```python
from build123d import *

# Parameters (mm, degrees)
EXTRUDE_1_DEPTH       = 2
HOLE_WIZARD_M81_D     = 8.4
HOLE_WIZARD_M81_DEPTH = 2
CHAMFER_1_SIZE        = 2


with BuildPart() as part:
    # Эскиз1 → Бобышка-Вытянуть1 (new body)
    with BuildSketch(Plane(origin=(0, 0, 0), x_dir=(1, 0, 0), z_dir=(0, 0, -1))):
        Polygon((0, 0), (0, 200), (100, 200), (100, 100), (50, 0), align=None)
    extrude(amount=EXTRUDE_1_DEPTH)

    # Отверстие с зазором M81
    with Locations(Plane(origin=(0, 0, -2), x_dir=(1, 0, 0), z_dir=(0, 0, -1))):
        with Locations((25, 175), (25, 125), (25, 75), (25, 25), (75, 175), (75, 125)):
            Hole(HOLE_WIZARD_M81_D / 2, depth=HOLE_WIZARD_M81_DEPTH)

    # Фаска1
    chamfer_1_edges = [part.edges().sort_by_distance(p)[0] for p in [
        (0, 0, -1),
        (0, -200, -1),
        (100, -200, -1),
    ]]
    chamfer(chamfer_1_edges, length=CHAMFER_1_SIZE)


solid = part.part
```
The model under review builds one solid part; all positions refer to its coordinate system, in mm. Round coordinates to 2 decimals unless told otherwise and drop trailing zeros. Loops run counter-clockwise (first coordinate to the right, second up) from the corner with the lowest first, then second, coordinate; pieces in that order, holes last. Notation, with made-up numbers: (47.5, 48.25) - (78.5, 48.25) arc R15 cw to (78.5, 65.25) - close; hole circle Ø5 at (71.5, -4.75). An arc over 180 degrees is marked (long way). Write each question's results on one line, items separated by ' | '. Start each with the question number.
Q1. Draft analysis for pull direction X (two halves, no side actions). For faces 1 (the flat face through (75.35, -50.7, -0.99)), 2 (the cylindrical face through (25.91, -70.9, -0.99)), 3 (the flat face through (51, -101, -2)), 4 (the cylindrical face through (28.3, -122.4, -1)), state which applies: pulls with the +X half, pulls with the -X half, needs draft (parallel to the pull), parting line crosses it, or undercut.
Q2. Take a section at C-C on x = 75. Give the boundary of the cut face in (y, z), plus the area to 3 significant figures.
Q3. Take a section at B-B on y = -175. Give the boundary of the cut face in (x, z), plus the area to 3 significant figures.
Q4. Wall thickness on line 1 along Y through (x, z) = (25, -0.2); line 2 along X through (y, z) = (-175, -1.5); line 3 along Y through (x, z) = (75, -1): over which ranges is each line inside the solid? List them lowest first. Write a range as [from, to].
Q5. Insertion check: P1, Ø5, axis at x = 25, y = -175, coming from the +Z side. The pin has a flat end and moves straight along its axis. Give the tip position at first contact, or say it passes through.
Q6. Take a section at D-D on y = -25. Give the boundary of the cut face in (x, z), plus the area to 3 significant figures.
Q7. Take a section at A-A on x = 25. Give the boundary of the cut face in (y, z).
Data:
1) face 1: pulls with the +X half | face 2: undercut | face 3: needs draft | face 4: undercut
2) outline: (-200, -2) - (-179.2, -2) - (-179.2, 0) - (-200, 0) - close; (-170.8, -2) - (-129.2, -2) - (-129.2, 0) - (-170.8, 0) - close; (-120.8, -2) - (-50, -2) - (-50, 0) - (-120.8, 0) - close | area: 266 mm²
3) outline: (0, -2) - (20.8, -2) - (20.8, 0) - (0, 0) - close; (29.2, -2) - (70.8, -2) - (70.8, 0) - (29.2, 0) - close; (79.2, -2) - (100, -2) - (100, 0) - (79.2, 0) - close | area: 166 mm²
4) line 1: y = [-200, -179.2], [-170.8, -129.2], [-120.8, -79.2], [-70.8, -29.2], [-20.8, 0] | line 2: x = [0, 20.8], [29.2, 70.8], [79.2, 100] | line 3: y = [-200, -179.2], [-170.8, -129.2], [-120.8, -50]
5) P1: passes through
6) outline: (0, -2) - (20.8, -2) - (20.8, 0) - (0, 0) - close; (29.2, -2) - (62.5, -2) - (62.5, 0) - (29.2, 0) - close | area: 108 mm²
7) outline: (-200, -2) - (-179.2, -2) - (-179.2, 0) - (-200, 0) - close; (-170.8, -2) - (-129.2, -2) - (-129.2, 0) - (-170.8, 0) - close; (-120.8, -2) - (-79.2, -2) - (-79.2, 0) - (-120.8, 0) - close; (-70.8, -2) - (-29.2, -2) - (-29.2, 0) - (-70.8, 0) - close; (-20.8, -2) - (0, -2) - (0, 0) - (-20.8, 0) - close
